```python
from build123d import *

# Parameters (mm, degrees)
SKETCH_1_W                = 120
SKETCH_1_H                = 105
EXTRUDE_1_DEPTH           = 10
HOLE_WIZARD_1_D           = 6.6
HOLE_WIZARD_1_CBORE_D     = 11
HOLE_WIZARD_1_CBORE_DEPTH = 6.8
HOLE_WIZARD_1_2_D         = 12
CUT_EXTRUDE_2_REACH       = 82.351
HOLE_WIZARD_M5_1_D        = 4.2
HOLE_WIZARD_M5_1_DEPTH    = 10.4
HOLE_WIZARD_M5_1_TIP      = 1.2618073
CHAMFER_1_SIZE            = 5


with BuildPart() as part:
    # 草图1 → 凸台-拉伸1 (new body)
    with BuildSketch(Plane(origin=(0, 0, 0), x_dir=(1, 0, 0), z_dir=(0, 1, 0))):
        Rectangle(SKETCH_1_W, SKETCH_1_H)
    extrude(amount=EXTRUDE_1_DEPTH)

    # Hole Wizard 1 (through all)
    with Locations(Plane(origin=(0, 0, 0), x_dir=(-1, 0, 0), z_dir=(0, -1, 0))):
        with Locations((39, -11.5), (-39, -11.5), (-39, 36.5), (39, 36.5)):
            CounterBoreHole(HOLE_WIZARD_1_D / 2, HOLE_WIZARD_1_CBORE_D / 2, HOLE_WIZARD_1_CBORE_DEPTH)

    # Hole Wizard 1 2 (through all)
    with Locations(Plane(origin=(0, 10, 0), x_dir=(1, 0, 0), z_dir=(0, 1, 0))):
        with Locations((0, 42.5)):
            Hole(HOLE_WIZARD_1_2_D / 2)

    # 草图7 → 切除-拉伸2 (cut, up to next)
    with BuildSketch(Plane(origin=(0, 10, 0), x_dir=(1, 0, 0), z_dir=(0, 1, 0)), mode=Mode.PRIVATE) as cut_extrude_2_sk1:
        with BuildLine():
            ThreePointArc((-37.401716164, -37.708239153), (-30.268782684, -40.66279694), (-22.905485492, -42.984435627))
            ThreePointArc((-22.905485492, -42.984435627), (-18.618878442, -40.509561892), (-21.093752176, -36.222954843))
            ThreePointArc((-21.093752176, -36.222954843), (-27.874641681, -34.084948594), (-34.443388332, -31.364084643))
            ThreePointArc((-34.443388332, -31.364084643), (-39.094629503, -33.056997982), (-37.401716164, -37.708239153))
        make_face()
    cut_extrude_2_tool1 = extrude(cut_extrude_2_sk1.sketch, amount=-CUT_EXTRUDE_2_REACH, mode=Mode.PRIVATE) & part.part
    # 草图7 → 切除-拉伸2 (cut, up to next)
    with BuildSketch(Plane(origin=(0, 10, 0), x_dir=(1, 0, 0), z_dir=(0, 1, 0)), mode=Mode.PRIVATE) as cut_extrude_2_sk2:
        with BuildLine():
            ThreePointArc((34.443388332, -31.364084643), (39.094629503, -33.056997982), (37.401716164, -37.708239153))
            ThreePointArc((37.401716164, -37.708239153), (30.268782684, -40.66279694), (22.905485492, -42.984435627))
            ThreePointArc((22.905485492, -42.984435627), (18.618878442, -40.509561892), (21.093752176, -36.222954843))
            ThreePointArc((21.093752176, -36.222954843), (27.874641681, -34.084948594), (34.443388332, -31.364084643))
        make_face()
    cut_extrude_2_tool2 = extrude(cut_extrude_2_sk2.sketch, amount=-CUT_EXTRUDE_2_REACH, mode=Mode.PRIVATE) & part.part
    add(cut_extrude_2_tool1.solids().sort_by_distance((-29.014889, 10, 37.217751))[0], mode=Mode.SUBTRACT)
    add(cut_extrude_2_tool2.solids().sort_by_distance((29.014889, 10, 37.217751))[0], mode=Mode.SUBTRACT)

    # M5 螺纹孔1
    with Locations(Plane(origin=(-19.270259274, 3.138381988, 52.5), x_dir=(1, 0, 0), z_dir=(0, 0, 1))):
        with Locations((-30.729740726, 1.861618012), (69.270259274, 1.861618012), (19.270259274, 1.861618012)):
            Hole(HOLE_WIZARD_M5_1_D / 2, depth=HOLE_WIZARD_M5_1_DEPTH)
            with Locations((0, 0, -(HOLE_WIZARD_M5_1_DEPTH + HOLE_WIZARD_M5_1_TIP / 2))):  # 118° drill point
                Cone(0, HOLE_WIZARD_M5_1_D / 2, HOLE_WIZARD_M5_1_TIP, mode=Mode.SUBTRACT)

    # 倒角1
    chamfer_1_edges = [part.edges().sort_by_distance(p)[0] for p in [
        (-60, 5, -52.5),
        (60, 5, -52.5),
    ]]
    chamfer(chamfer_1_edges, length=CHAMFER_1_SIZE)


solid = part.part
```
Model file for the job. Use its own axes, mm. A direction names the side the tool comes from. Coordinates: 2 decimals unless noted, no trailing zeros. Write each loop counter-clockwise with the first axis right and the second up, starting at its lowest first coordinate (ties: lowest second). Pieces come first, ordered by that corner, then holes. Notation, with made-up numbers: (72, -31) - (84, -31) arc R15 cw to (84, -18) - close; hole circle Ø1 at (41.25, 70.25). An arc over 180 degrees is marked (long way). Use a Markdown table: item, result. Add a question column.
Item 1: Drill centre lines: line 1 along X through (y, z) = (5, 45.25); line 2 along X through (y, z) = (2.25, -42.5); line 3 along X through (y, z) = (5.5, -39.5). Where is each one in solid material? Low to high.
Item 2: Band-saw the part on C-C, the plane z = -44.5. Write the cut outline in (x, y).
Item 3: Band-saw the part on A-A, the plane y = 1.5. Write the cut outline in (x, z).
Item 4: Band-saw the part on B-B, the plane x = 4.5. Write the cut outline in (y, z).
Item 5: 3-axis set-ups, long thin cutter, end or side, ignore diameter. For faces 1 (the face through (-27.78, 5.07, 34.12)), 2 (the face through (43.4, 3.4, 14.8)), 3 (the face through (-1, 5, -52.5)), 4 (the face through (47.997, 5.631, 47.227)), 5 (the face through (-1, 10, -1)): which of +Z, -Z, +X, -X, +Y, -Y reach the whole face in a straight line?
Item 6: Two-plate mould, pull along Y, no slides. Class faces 6 (the face through (-52.003, 5.631, 47.227)), 7 (the face through (-39, 6.8, -33)), 8 (the face through (-0.8, 2.7, 52.5)): pulls with the +Y half, pulls with the -Y half, needs draft (parallel to the pull), parting line crosses it, or undercut.
Item 7: Drop flat-ended pins along their axis: pin 1 (3.5 mm diameter, centred on x = -40, z = 12, fed in from -Y); pin 2 (3.5 mm diameter, centred on x = -41, z = -34, fed in from -Y). Give the stop position or say it passes through.
A:
| question | item | result |
|---|---|---|
| 1 | line 1 | x = -60 to -52.1, -47.9 to -2.1, 2.1 to 47.9, 52.1 to 60 |
| 1 | line 2 | x = -60 to -6, 6 to 60 |
| 1 | line 3 | x = -60 to -43.61, -34.39 to -5.2, 5.2 to 34.39, 43.61 to 60 |
| 2 | outline | (-60, 0) - (-5.66, 0) - (-5.66, 10) - (-60, 10) - close; (5.66, 0) - (60, 0) - (60, 10) - (5.66, 10) - close |
| 3 | outline | (-60, -47.5) - (-55, -52.5) - (55, -52.5) - (60, -47.5) - (60, 52.5) - (-60, 52.5) - close; hole circle Ø11 at (-39, -36.5); hole circle Ø11 at (-39, 11.5); hole (-37.4, 37.71) arc R3.5 ccw to (-34.44, 31.36) arc R81.5 cw to (-21.09, 36.22) arc R3.5 ccw to (-22.91, 42.98) arc R88.5 ccw to start; hole circle Ø12 at (0, -42.5); hole (21.09, 36.22) arc R81.5 cw to (34.44, 31.36) arc R3.5 ccw to (37.4, 37.71) arc R88.5 ccw to (22.91, 42.98) arc R3.5 ccw to start; hole circle Ø11 at (39, -36.5); hole circle Ø11 at (39, 11.5) |
| 4 | outline | (0, -52.5) - (10, -52.5) - (10, -46.47) - (0, -46.47) - close; (0, -38.53) - (10, -38.53) - (10, 52.5) - (0, 52.5) - close |
| 5 | face 1 | +Y, -Y |
| 5 | face 2 | -Y |
| 5 | face 3 | -Z, +X, -X, +Y, -Y |
| 5 | face 4 | +Z |
| 5 | face 5 | +Z, -Z, +X, -X, +Y |
| 6 | face 6 | undercut |
| 6 | face 7 | pulls with the -Y half |
| 6 | face 8 | needs draft |
| 7 | pin 1 | passes through |
| 7 | pin 2 | stops at y = 6.8 |
